For this review, use the dimensioned drawing (mm, ordinates from the lowest corner) and the shaded views. A direction names the side the tool comes from. Coordinates: 2 decimals unless noted, no trailing zeros. Write each loop counter-clockwise with the first axis right and the second up, starting at its lowest first coordinate (ties: lowest second). Pieces come first, ordered by that corner, then holes.
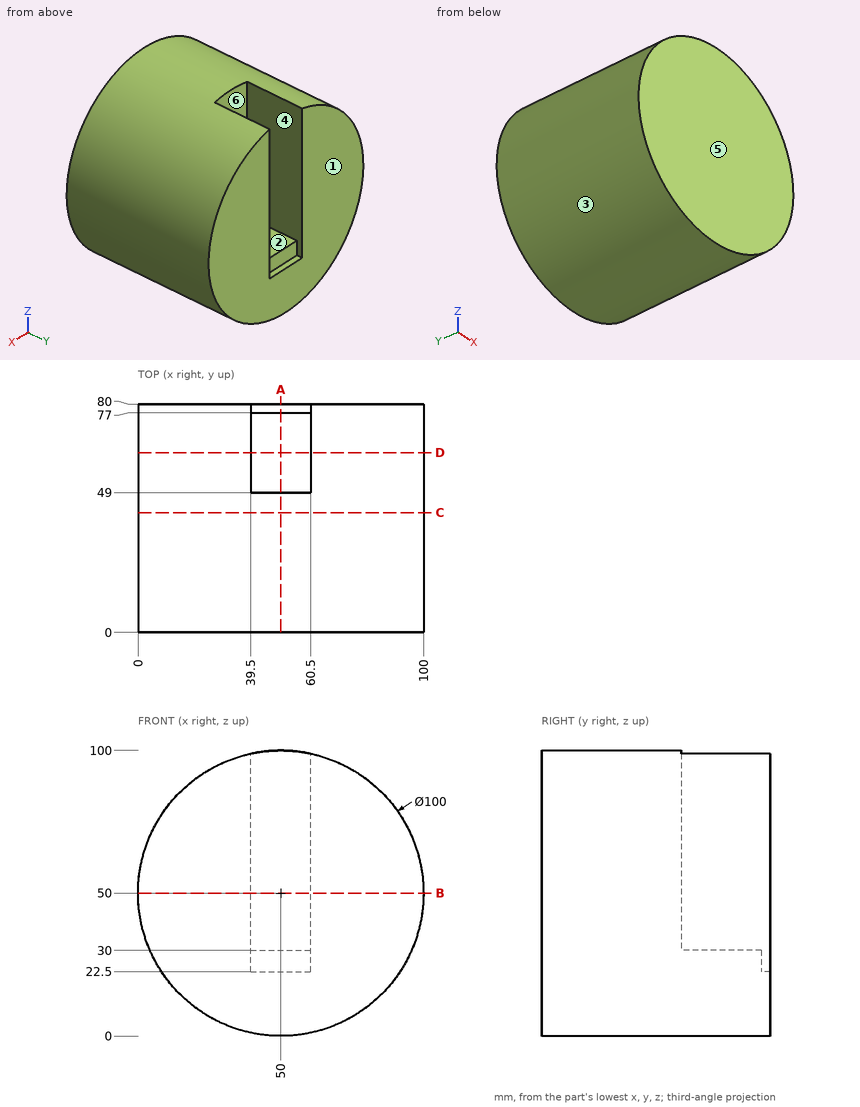
(1) Insertion check: pin 1 Ø12 at (x, z) = (70, 41) entering from -Y; pin 2 Ø9.5 at (y, z) = (63.5, 45.5) entering from -X; pin 3 Ø3 at (x, y) = (29, 69.5) entering from -Z; pin 4 Ø2.5 at (x, y) = (54.5, 78) entering from +Z. Each pin has a flat end and moves straight along its axis. Give the tip position at first contact, or say it passes through.
(2) Consider section B-B (z = 50). Give the boundary of the cut face in (x, y), plus the area to 3 significant figures.
(3) Wall thickness on line 1 (X direction, y = 70.5, z = 58); line 2 (X direction, y = 60.5, z = 36); line 3 (Y direction, x = 53, z = 72.5): over which ranges is each line inside the solid? List them lowest first.
(4) Consider section D-D (y = 63). Give the boundary of the cut face in (x, z), plus the area to 3 significant figures.
(5) Consider section C-C (y = 42). Give the boundary of the cut face in (x, z).
(6) Consider section A-A (x = 50). Give the boundary of the cut face in (y, z).
(7) For the marked faces 5 and 6, list the 3-axis set-ups (+Z, -Z, +X, -X, +Y, -Y) from which the entire face can be reached by the end or side of a thin tool; tool diameter is ignored.
(8) Mouldability with a two-part tool opening along X and no side actions: class the marked faces 1, 2, 3 and 4 as +X half, -X half, draft (parallel to the pull), parting line (faces both ways), or undercut.
Results:
1. pin 1: stops at y = 0
1. pin 2: stops at x = 0
1. pin 3: stops at z = 3.96
1. pin 4: stops at z = 30
2. outline: (0, 0) - (100, 0) - (100, 80) - (60.5, 80) - (60.5, 49) - (39.5, 49) - (39.5, 80) - (0, 80) - close
2. area: 7,350 mm2
3. line 1: x = 0.64 to 39.5, 60.5 to 99.36
3. line 2: x = 2 to 39.5, 60.5 to 98
3. line 3: y = 0 to 49
4. outline: (39.5, 30) - (39.5, 98.89) arc R50 ccw (long way) to (60.5, 98.89) - (60.5, 30) - close
4. area: 6,390 mm2
5. outline: circle Ø100 at (50, 50)
6. outline: (0, 0) - (80, 0) - (80, 22.5) - (77, 22.5) - (77, 30) - (49, 30) - (49, 100) - (0, 100) - close
7. face 5: +Z, -Z, +X, -X, -Y
7. face 6: +Z, +Y
8. face 1: draft
8. face 2: undercut
8. face 3: parting line
8. face 4: undercut
